```python
from build123d import *

# Parameters (mm, degrees)
CROQUIS1_W              = 30
CROQUIS1_H              = 30
CROQUIS1_W_2            = 24
CROQUIS1_H_2            = 24
SALIENTE_EXTRUIR1_DEPTH = 50
CROQUIS2_W              = 30
CROQUIS2_H              = 30
SALIENTE_EXTRUIR2_DEPTH = 2
CROQUIS6_W              = 30
CROQUIS6_H              = 4.83764523
SALIENTE_EXTRUIR4_DEPTH = 40
CROQUIS7_R              = 5.3
CROQUIS7_R_2            = 1.95
CORTAR_EXTRUIR2_DEPTH   = 40
REDONDEO1_R             = 2


with BuildPart() as part:
    # Croquis1 → Saliente-Extruir1 (new body)
    with BuildSketch(Plane(origin=(0, 0, 0), x_dir=(1, 0, 0), z_dir=(0, 1, 0))):
        Rectangle(CROQUIS1_W, CROQUIS1_H)
        Rectangle(CROQUIS1_W_2, CROQUIS1_H_2, mode=Mode.SUBTRACT)
    extrude(amount=SALIENTE_EXTRUIR1_DEPTH)

    # Croquis2 → Saliente-Extruir2 (add)
    with BuildSketch(Plane(origin=(0, 50, 0), x_dir=(1, 0, 0), z_dir=(0, 1, 0))):
        Rectangle(CROQUIS2_W, CROQUIS2_H)
    extrude(amount=SALIENTE_EXTRUIR2_DEPTH)

    # Croquis6 → Saliente-Extruir4 (add)
    with BuildSketch(Plane(origin=(0, 0, -15), x_dir=(-1, 0, 0), z_dir=(0, 0, -1))):
        with Locations((0, 49.581177385)):
            Rectangle(CROQUIS6_W, CROQUIS6_H)
    extrude(amount=SALIENTE_EXTRUIR4_DEPTH)

    # Croquis7 → Cortar-Extruir2 (cut)
    with BuildSketch(Plane(origin=(0, 52, 0), x_dir=(1, 0, 0), z_dir=(0, 1, 0))):
        with Locations((0, 41.634609849)):
            Circle(CROQUIS7_R)
        with Locations((7.424621202, 49.059231051)):
            Circle(CROQUIS7_R_2)
        with Locations((7.424621202, 34.209988647)):
            Circle(CROQUIS7_R_2)
        with Locations((-7.424621202, 34.209988647)):
            Circle(CROQUIS7_R_2)
        with Locations((-7.424621202, 49.059231051)):
            Circle(CROQUIS7_R_2)
    extrude(amount=-CORTAR_EXTRUIR2_DEPTH, mode=Mode.SUBTRACT)

    # Redondeo1
    redondeo1_edges = [part.edges().sort_by_distance(p)[0] for p in [
        (-15, 26, 15),
        (15, 26, 15),
        (15, 23.581177385, -15),
        (-15, 23.581177385, -15),
        (-12, 25, 12),
        (-12, 25, -12),
        (12, 25, 12),
        (12, 25, -12),
    ]]
    fillet(redondeo1_edges, radius=REDONDEO1_R)


solid = part.part
```
Could you check a few things on this model? Use its own coordinates, in mm. A direction names the side the tool comes from. Round coordinates to 2 decimals unless told otherwise and drop trailing zeros. Loops run counter-clockwise (first coordinate to the right, second up) from the corner with the lowest first, then second, coordinate; pieces in that order, holes last. Notation, with made-up numbers: (56, -1.5) - (106, -1.5) arc R8 cw to (106, 9.5) - close; hole circle Ø7 at (-6.5, -16). An arc over 180 degrees is marked (long way). Answer in a Markdown table with one row per item. Add a question column.
(1) If we mould it in two halves opening along Z, with no side actions, what happens to faces 4 (the face through (0, 50, 0)), 5 (the face through (0, 26, 15)), 6 (the face through (-15, 26, -5)), 7 (the face through (-14.4, 23.25, -14.43))? For each: pulls with the +Z half, pulls with the -Z half, needs draft (parallel to the pull), parting line crosses it, or undercut.
(2) I'm going to push flat-ended pins straight in: pin 1 (10 mm diameter, centred on x = 7.5, y = 36, fed in from -Z); pin 2 (12 mm diameter, centred on x = -2.5, z = 2.5, fed in from -Y); pin 3 (9 mm diameter, centred on x = 3, z = -28, fed in from -Y). Where does each tip first touch, or does it pass through?
(3) If we section it at D-D (z = 0.5): Please give me the cut outline in (x, y).
(4) If we section it at C-C (z = -43.5): Please give me the cut outline in (x, y).
(5) For faces 1 (the face through (11.43, 25.35, -11.4)), 2 (the face through (0, 23, -15)), 3 (the face through (-14, 0, 0)), which set-ups out of +Z, -Z, +X, -X, +Y, -Y let a thin tool reach every point of the face, with its end or its side?
(6) If we section it at B-B (x = 0): Please give me the cut outline in (y, z), plus the area to 3 significant figures.
(7) If we section it at A-A (y = 4): Please give me the cut outline in (x, z).
(8) I need wall thicknesses on line 1 along Z through (x, y) = (5.75, 32); line 2 along Y through (x, z) = (10.5, -1). Which ranges of each line are inside material? Lowest first, please.
Model answer:
| question | item | result |
|---|---|---|
| 1 | face 4 | undercut |
| 1 | face 5 | pulls with the +Z half |
| 1 | face 6 | needs draft |
| 1 | face 7 | pulls with the -Z half |
| 2 | pin 1 | stops at z = -15 |
| 2 | pin 2 | stops at y = 50 |
| 2 | pin 3 | stops at y = 47.16 |
| 3 | outline | (-15, 0) - (-12, 0) - (-12, 50) - (12, 50) - (12, 0) - (15, 0) - (15, 52) - (-15, 52) - close |
| 4 | outline | (-15, 47.16) - (-4.96, 47.16) - (-4.96, 52) - (-15, 52) - close; (4.96, 47.16) - (15, 47.16) - (15, 52) - (4.96, 52) - close |
| 5 | face 1 | -Y |
| 5 | face 2 | -Z, +X, -X, -Y |
| 5 | face 3 | +Z, -Z, +X, -X, -Y |
| 6 | outline | (0, -15) - (47.16, -15) - (47.16, -36.33) - (52, -36.33) - (52, 15) - (0, 15) - (0, 12) - (50, 12) - (50, -12) - (0, -12) - close; (47.16, -55) - (52, -55) - (52, -46.93) - (47.16, -46.93) - close |
| 6 | area | 502 mm² |
| 7 | outline | (-15, -13) arc R2 ccw to (-13, -15) - (13, -15) arc R2 ccw to (15, -13) - (15, 13) arc R2 ccw to (13, 15) - (-13, 15) arc R2 ccw to (-15, 13) - close; hole (-12, -10) arc R2 ccw to (-10, -12) - (10, -12) arc R2 ccw to (12, -10) - (12, 10) arc R2 ccw to (10, 12) - (-10, 12) arc R2 ccw to (-12, 10) - close |
| 8 | line 1 | z = -15 to -12, 12 to 15 |
| 8 | line 2 | y = 50 to 52 |
